The listing builds one solid part. Answer for the finished solid, in the listing's coordinates (mm). Coordinates: 2 decimals unless noted, no trailing zeros. Order: outer loops, then holes, each group sorted by start corner. A loop starts at its lowest first (then second) coordinate and runs counter-clockwise, first axis right, second up. Notation, with made-up numbers: (-34, 81) -> (-7, 81) arc R35 ccw to (-7, 114) -> close; hole circle Ø2 at (18.25, 58.25). An arc over 180 degrees is marked (long way). Answer in a Markdown table with one row per item.
```python
from build123d import *

# Parameters (mm, degrees)
SKETCH1_W           = 116
SKETCH1_H           = 20
BOSS_EXTRUDE2_DEPTH = 5
SKETCH4_R           = 1
CUT_EXTRUDE1_DEPTH  = 10
SKETCH6_R           = 1
CUT_EXTRUDE2_DEPTH  = 5
SKETCH7_R           = 1
CUT_EXTRUDE3_DEPTH  = 6
SKETCH8_R           = 1
CUT_EXTRUDE4_DEPTH  = 6


with BuildPart() as part:
    # Sketch1 → Boss-Extrude2 (new body)
    with BuildSketch(Plane.XY):
        Rectangle(SKETCH1_W, SKETCH1_H)
    extrude(amount=BOSS_EXTRUDE2_DEPTH)

    # Sketch4 → Cut-Extrude1 (cut)
    with BuildSketch(Plane(origin=(58, 0, 0), x_dir=(0, 0, -1), z_dir=(1, 0, 0))):
        with Locations((-2.5, -5.12)):
            Circle(SKETCH4_R)
        with Locations((-2.5, 5.12)):
            Circle(SKETCH4_R)
    extrude(amount=-CUT_EXTRUDE1_DEPTH, mode=Mode.SUBTRACT)

    # Sketch6 → Cut-Extrude2 (cut)
    with BuildSketch(Plane.ZY.offset(58)):
        with Locations((2.5, 5)):
            Circle(SKETCH6_R)
        with Locations((2.5, -5)):
            Circle(SKETCH6_R)
    extrude(amount=-CUT_EXTRUDE2_DEPTH, mode=Mode.SUBTRACT)

    # Sketch7 → Cut-Extrude3 (cut, through all)
    with BuildSketch(Plane(origin=(0, 0, 0), x_dir=(-1, 0, 0), z_dir=(0, 0, -1))):
        with Locations((-45, 5)):
            Circle(SKETCH7_R)
        with Locations((-45, -5)):
            Circle(SKETCH7_R)
        with Locations((45, 5)):
            Circle(SKETCH7_R)
        with Locations((45, -5)):
            Circle(SKETCH7_R)
    extrude(amount=-CUT_EXTRUDE3_DEPTH, mode=Mode.SUBTRACT)

    # Sketch8 → Cut-Extrude4 (cut, through all)
    with BuildSketch(Plane(origin=(0, 0, 0), x_dir=(-1, 0, 0), z_dir=(0, 0, -1))):
        with Locations((19.8, -8)):
            Circle(SKETCH8_R)
        with Locations((19.8, -2)):
            Circle(SKETCH8_R)
        with Locations((8.8, -2)):
            Circle(SKETCH8_R)
        with Locations((8.8, -8)):
            Circle(SKETCH8_R)
    extrude(amount=-CUT_EXTRUDE4_DEPTH, mode=Mode.SUBTRACT)


solid = part.part
```
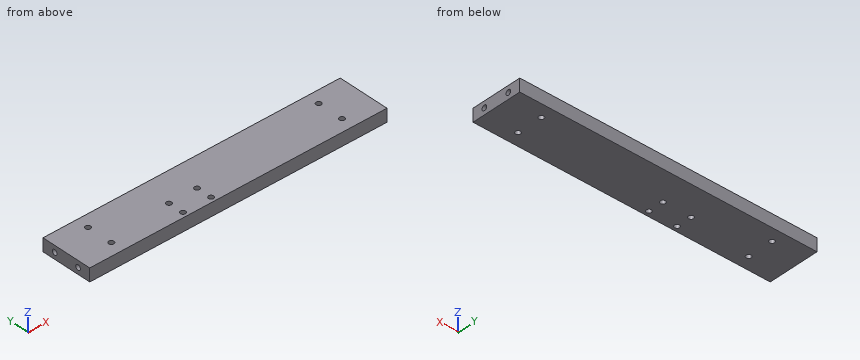
(1) A cutting plane is placed at B-B, the plane y = -8. Determine the outline of the cut face in (x, z).
Check values:
| item | result |
|---|---|
| outline | (-58, 0) -> (-20.8, 0) -> (-20.8, 5) -> (-58, 5) -> close; (-18.8, 0) -> (-9.8, 0) -> (-9.8, 5) -> (-18.8, 5) -> close; (-7.8, 0) -> (58, 0) -> (58, 5) -> (-7.8, 5) -> close |
(2) A cutting plane is placed at C-C, the plane z = 2.5. Count the separate pieces of the cut face and the enclosed holes in it, then the cut area to 3 significant figures.
Check values:
| item | result |
|---|---|
| separate pieces | 1 |
| enclosed holes | 8 |
| area | 2,230 mm² |
(3) Flat-ended cylindrical pins translate along their axes: pin 1 (1.6 mm diameter, centred on x = 45, y = -5, fed in from +Z) (3 decimals); pin 2 (1.6 mm diameter, centred on y = -5, z = 2.5, fed in from +X); pin 3 (0.6 mm diameter, centred on y = 5, z = 2.5, fed in from -X). Find the tip coordinate at first contact, or state that the pin passes through.
Check values:
| item | result |
|---|---|
| pin 1 | through |
| pin 2 | x = 48 |
| pin 3 | x = -53 |
(4) Find the intervals of material crossed by line 1 along Y through (x, z) = (-8.8, 2.75); line 2 along Y through (x, z) = (-45, 2.6); line 3 along X through (y, z) = (-8.75, 0.9), in increasing order. Write a range as from..to.
Check values:
| item | result |
|---|---|
| line 1 | -10..-9, -7..-3, -1..10 |
| line 2 | -10..-6, -4..4, 6..10 |
| line 3 | -58..-20.46, -19.14..-9.46, -8.14..58 |
(5) A cutting plane is placed at A-A, the plane x = 45. Determine the outline of the cut face in (y, z), then the cut area to 3 significant figures.
Check values:
| item | result |
|---|---|
| outline | (-10, 0) -> (-6, 0) -> (-6, 5) -> (-10, 5) -> close; (-4, 0) -> (4, 0) -> (4, 5) -> (-4, 5) -> close; (6, 0) -> (10, 0) -> (10, 5) -> (6, 5) -> close |
| area | 80.0 mm² |
